Geometry: final body of the model. Coordinates: model frame, mm. Face numbers are marked on the shaded views. A direction names the side the tool comes from. Give positions to 0.01 mm unless a question says otherwise; leave off trailing zeros. Loops run counter-clockwise (first coordinate to the right, second up) from the corner with the lowest first, then second, coordinate; pieces in that order, holes last. Notation, with made-up numbers: (46.5, -30) -> (74.5, -30) arc R22 ccw to (74.5, -8) -> close; hole circle Ø5 at (66, -24.5). An arc over 180 degrees is marked (long way). One line per question, with ' | ' between items. Start each with the question number.
Item 1: Set-up query: the marked faces 1, 2 and 3. Return all of +Z, -Z, +X, -X, +Y, -Y with unobstructed straight access to the full face (end or side cutting, diameter ignored); none if empty.
Item 2: Section B-B on z = 0.5. Return loops of the section in (x, y), then the cut area to 3 significant figures.
Item 3: Mould query, pull axis Z, two halves, no side actions, for the marked faces 4, 5, 6 and 7. Classes: released by +Z, released by -Z, zero draft, split by the parting line, or undercut.
Item 4: Section A-A on x = 0. Return loops of the section in (y, z), then the cut area to 3 significant figures.
Item 5: Material intervals for line 1 along Z through (x, y) = (0, -1.85); line 2 along Y through (x, z) = (-2.5, -1.5); line 3 along X through (y, z) = (-8, -7.25), sorted ascending. Write a range as [from, to].
Item 6: Section C-C on y = -9. Return loops of the section in (x, z), then the cut area to 3 significant figures.
Item 7: Section D-D on z = -6. Return loops of the section in (x, y), then the cut area to 3 significant figures.
Item 8: Pin query (flat end, axial travel): P1, Ø3.5, axis at x = 0, z = -5.5, coming from the -Y side; P2, Ø6, axis at x = 0, y = -9, coming from the -Z side; P3, Ø5, axis at x = 0, z = -5.5, coming from the +Y side; P4, Ø2.5, axis at x = 0, z = -5.5, coming from the -Y side (3 decimals). Return the tip coordinate at first contact, or that it passes through.
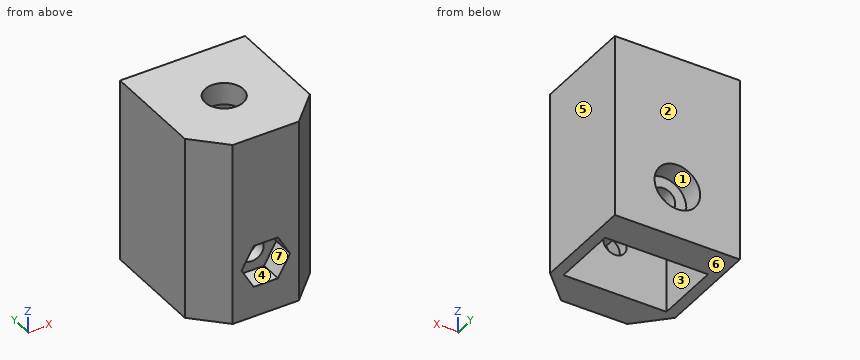
from build123d import *

# Parameters (mm, degrees)
F0_W      = 17
F0_H      = 25
F1_DEPTH  = 18
F2_W      = 14
F2_H      = 9
F3_DEPTH  = 22
F4_R      = 1.6
F5_DEPTH  = 25
F6_R      = 2.6
F7_DEPTH  = 25
F8_R      = 3.1
F9_DEPTH  = 3
F11_DEPTH = 3
F12_SIZE  = 4


with BuildPart() as f1:
    # F0 (on Front) → F1 (new body)
    with BuildSketch(Plane.XZ):
        Rectangle(F0_W, F0_H)
    extrude(amount=F1_DEPTH)

    # F2 (on face) → F3 (cut, through all)
    with BuildSketch(Plane(origin=(0, 0, -12.5), x_dir=(1, 0, 0), z_dir=(0, 0, -1))):
        with Locations((0, 9)):
            Rectangle(F2_W, F2_H)
    extrude(amount=-F3_DEPTH, mode=Mode.SUBTRACT)

    # F4 (on face) → F5 (cut)
    with BuildSketch(Plane.XZ.offset(18)):
        with Locations((0, -5.5)):
            Circle(F4_R)
    extrude(amount=-F5_DEPTH, mode=Mode.SUBTRACT)

    # F6 (on face) → F7 (cut)
    with BuildSketch(Plane.XY.offset(12.5)):
        with Locations((0, -9)):
            Circle(F6_R)
    extrude(amount=-F7_DEPTH, mode=Mode.SUBTRACT)

    # F8 (on face) → F9 (cut)
    with BuildSketch(Plane(origin=(0, 0, 0), x_dir=(-1, 0, 0), z_dir=(0, 1, 0))):
        with Locations((0, -5.5)):
            Circle(F8_R)
    extrude(amount=-F9_DEPTH, mode=Mode.SUBTRACT)

    # F10 (on face) → F11 (cut)
    with BuildSketch(Plane.XZ.offset(18)):
        Polygon((-1.65, -8.3578838325), (1.65, -8.3578838325), (3.3, -5.5), (1.65, -2.6421161675), (-1.65, -2.6421161675), (-3.3, -5.5), align=None)
    extrude(amount=-F11_DEPTH, mode=Mode.SUBTRACT)

    # F12
    f12_edges = [f1.edges().sort_by_distance(p)[0] for p in [
        (8.5, -18, 0),
        (-8.5, -18, 0),
    ]]
    chamfer(f12_edges, length=F12_SIZE)


solid = f1.part
Result sheet:
1) face 1: +Y | face 2: +Z, -Z, +X, -X, +Y | face 3: -Z
2) outline: (-8.5, -14) -> (-4.5, -18) -> (4.5, -18) -> (8.5, -14) -> (8.5, 0) -> (-8.5, 0) -> close; hole (-7, -13.5) -> (7, -13.5) -> (7, -4.5) -> (-7, -4.5) -> close | area: 164 mm²
3) face 4: undercut | face 5: zero draft | face 6: released by -Z | face 7: undercut
4) outline: (-18, -12.5) -> (-13.5, -12.5) -> (-13.5, -7.1) -> (-15, -7.1) -> (-15, -8.36) -> (-18, -8.36) -> close; (-18, -2.64) -> (-15, -2.64) -> (-15, -3.9) -> (-13.5, -3.9) -> (-13.5, 9.5) -> (-11.6, 9.5) -> (-11.6, 12.5) -> (-18, 12.5) -> close; (-6.4, 9.5) -> (-4.5, 9.5) -> (-4.5, -3.9) -> (-3, -3.9) -> (-3, -2.4) -> (0, -2.4) -> (0, 12.5) -> (-6.4, 12.5) -> close; (-4.5, -12.5) -> (0, -12.5) -> (0, -8.6) -> (-3, -8.6) -> (-3, -7.1) -> (-4.5, -7.1) -> close | area: 191 mm²
5) line 1: z = [-12.5, -8.6], [-2.4, 12.5] | line 2: y = [-18, -13.5], [-4.5, 0] | line 3: x = [-8.5, -7], [7, 8.5]
6) outline: (-8.5, -12.5) -> (-7, -12.5) -> (-7, 9.5) -> (-2.6, 9.5) -> (-2.6, 12.5) -> (-8.5, 12.5) -> close; (2.6, 9.5) -> (7, 9.5) -> (7, -12.5) -> (8.5, -12.5) -> (8.5, 12.5) -> (2.6, 12.5) -> close | area: 101 mm²
7) outline: (-8.5, -14) -> (-4.5, -18) -> (-3.01, -18) -> (-3.01, -15) -> (-1.52, -15) -> (-1.52, -13.5) -> (-7, -13.5) -> (-7, -4.5) -> (-1.52, -4.5) -> (-1.52, -3) -> (-3.06, -3) -> (-3.06, 0) -> (-8.5, 0) -> close; (1.52, -15) -> (3.01, -15) -> (3.01, -18) -> (4.5, -18) -> (8.5, -14) -> (8.5, 0) -> (3.06, 0) -> (3.06, -3) -> (1.52, -3) -> (1.52, -4.5) -> (7, -4.5) -> (7, -13.5) -> (1.52, -13.5) -> close | area: 118 mm²
8) P1: stops at y = -15 | P2: stops at z = 9.5 | P3: stops at y = -3 | P4: passes through
